```python
from build123d import *

# Parameters (mm, degrees)
SKETCH1_W           = 140
SKETCH1_H           = 25
BOSS_EXTRUDE1_DEPTH = 25
CUT_EXTRUDE1_DEPTH  = 25
CUT_EXTRUDE13_DEPTH = 3
SKETCH9_W           = 80
SKETCH9_H           = 18.70062617
CUT_EXTRUDE14_DEPTH = 3


with BuildPart() as part:
    # Sketch1 → Boss-Extrude1 (new body)
    with BuildSketch(Plane(origin=(0, 0, 0), x_dir=(1, 0, 0), z_dir=(0, 1, 0))):
        Rectangle(SKETCH1_W, SKETCH1_H)
    extrude(amount=BOSS_EXTRUDE1_DEPTH)

    # Sketch5 → Cut-Extrude1 (cut)
    with BuildSketch(Plane.XY.offset(12.5)):
        with BuildLine():
            add(Edge.make_bspline(
                [(0, 23), (15, 23), (30, 23.367346939)],
                knots=[0.5, 0.5, 0.5, 0.714285714, 0.714285714, 0.714285714], degree=2))
            add(Edge.make_bspline(
                [(30, 23.367346939), (50, 23.857142857), (70, 25)],
                knots=[0.714285714, 0.714285714, 0.714285714, 1, 1, 1], degree=2))
            Line((70, 25), (30, 25))
            Line((30, 25), (0, 25))
            Line((0, 25), (0, 23))
        make_face()
        with BuildLine():
            add(Edge.make_bspline(
                [(-50, 24.020408163), (-25, 23), (0, 23)],
                knots=[0.142857143, 0.142857143, 0.142857143, 0.5, 0.5, 0.5], degree=2))
            Line((0, 23), (0, 25))
            Line((0, 25), (-50, 25))
            Line((-50, 25), (-70, 25))
            add(Edge.make_bspline(
                [(-70, 25), (-60, 24.428571429), (-50, 24.020408163)],
                knots=[0, 0, 0, 0.142857143, 0.142857143, 0.142857143], degree=2))
        make_face()
        with BuildLine():
            Line((30, 19.867346939), (30, 23.367346939))
            add(Edge.make_bspline(
                [(0, 23), (15, 23), (30, 23.367346939)],
                knots=[0.5, 0.5, 0.5, 0.714285714, 0.714285714, 0.714285714], degree=2))
            Line((0, 23), (0, 19.5))
            add(Edge.make_bspline(
                [(0, 19.5), (14.999250637, 19.500030588), (30, 19.867346939)],
                knots=[0.625031228, 0.625031228, 0.625031228, 1, 1, 1], degree=2))
        make_face()
        with BuildLine():
            Line((0, 19.5), (0, 23))
            add(Edge.make_bspline(
                [(-50, 24.020408163), (-25, 23), (0, 23)],
                knots=[0.142857143, 0.142857143, 0.142857143, 0.5, 0.5, 0.5], degree=2))
            Line((-50, 24.020408163), (-50, 21.5))
            Line((-50, 21.5), (-50, 20.520408163))
            add(Edge.make_bspline(
                [(-50, 20.520408163), (-25.002082119, 19.499949013), (0, 19.5)],
                knots=[0, 0, 0, 0.625031228, 0.625031228, 0.625031228], degree=2))
        make_face()
        with BuildLine():
            Line((0, 0), (0, 3.5))
            add(Edge.make_bspline(
                [(-50, 4.813033374), (-25.004215516, 3.554754755), (0, 3.5)],
                knots=[0, 0, 0, 0.625063216, 0.625063216, 0.625063216], degree=2))
            Line((-50, 4.813033374), (-50, 1.020408163))
            add(Edge.make_bspline(
                [(-50, 1.020408163), (-25, 0), (0, 0)],
                knots=[0.142857143, 0.142857143, 0.142857143, 0.5, 0.5, 0.5], degree=2))
        make_face()
        with BuildLine():
            Line((30, 0.367346939), (30, 3.867346939))
            add(Edge.make_bspline(
                [(0, 3.5), (14.998483233, 3.467156007), (30, 3.867346939)],
                knots=[0.625063216, 0.625063216, 0.625063216, 1, 1, 1], degree=2))
            Line((0, 3.5), (0, 0))
            add(Edge.make_bspline(
                [(0, 0), (15, 0), (30, 0.367346939)],
                knots=[0.5, 0.5, 0.5, 0.714285714, 0.714285714, 0.714285714], degree=2))
        make_face()
        with BuildLine():
            Line((70, 0), (70, 2))
            add(Edge.make_bspline(
                [(30, 0.367346939), (50, 0.857142857), (70, 2)],
                knots=[0.714285714, 0.714285714, 0.714285714, 1, 1, 1], degree=2))
            add(Edge.make_bspline(
                [(0, 0), (15, 0), (30, 0.367346939)],
                knots=[0.5, 0.5, 0.5, 0.714285714, 0.714285714, 0.714285714], degree=2))
            Line((0, 0), (70, 0))
        make_face()
        with BuildLine():
            Line((-70, 0), (0, 0))
            add(Edge.make_bspline(
                [(-50, 1.020408163), (-25, 0), (0, 0)],
                knots=[0.142857143, 0.142857143, 0.142857143, 0.5, 0.5, 0.5], degree=2))
            add(Edge.make_bspline(
                [(-70, 2), (-60, 1.428571429), (-50, 1.020408163)],
                knots=[0, 0, 0, 0.142857143, 0.142857143, 0.142857143], degree=2))
            Line((-70, 2), (-70, 0))
        make_face()
    extrude(amount=-CUT_EXTRUDE1_DEPTH, mode=Mode.SUBTRACT)

    # Sketch6 → Cut-Extrude13 (cut)
    with BuildSketch(Plane.XY.offset(12.5)):
        with BuildLine():
            Line((30, 1.485887188), (30, 3.867346939))
            add(Edge.make_bspline(
                [(-50, 4.813033374), (-10.010789538, 2.799991192), (30, 3.867346939)],
                knots=[0, 0, 0, 1, 1, 1], degree=2))
            Line((-50, 4.813033374), (-50, 1.485887188))
            Line((-50, 1.485887188), (30, 1.485887188))
        make_face()
        with BuildLine():
            Line((-50, 20.520408163), (-50, 4.813033374))
            add(Edge.make_bspline(
                [(-50, 4.813033374), (-10.010789538, 2.799991192), (30, 3.867346939)],
                knots=[0, 0, 0, 1, 1, 1], degree=2))
            Line((30, 3.867346939), (30, 19.867346939))
            add(Edge.make_bspline(
                [(30, 19.867346939), (-10.005329691, 18.887755097), (-50, 20.520408163)],
                knots=[0, 0, 0, 1, 1, 1], degree=2))
        make_face()
        Polygon((-50, 20.520408163), (30, 19.867346939), (30, 20.995155466), (30, 21.46990277), (-50, 21.46990277), align=None)
        with BuildLine():
            Line((-50, 20.520408163), (30, 19.867346939))
            add(Edge.make_bspline(
                [(30, 19.867346939), (-10.005329691, 18.887755097), (-50, 20.520408163)],
                knots=[0, 0, 0, 1, 1, 1], degree=2))
        make_face()
    extrude(amount=-CUT_EXTRUDE13_DEPTH, mode=Mode.SUBTRACT)

    # Sketch9 → Cut-Extrude14 (cut)
    with BuildSketch(Plane(origin=(0, 0, -12.5), x_dir=(-1, 0, 0), z_dir=(0, 0, -1))):
        with Locations((10, 12.267033854)):
            Rectangle(SKETCH9_W, SKETCH9_H)
    extrude(amount=-CUT_EXTRUDE14_DEPTH, mode=Mode.SUBTRACT)


solid = part.part
```
Geometry: final body of the model. Coordinates: model frame, mm. A direction names the side the tool comes from. Give positions to 0.01 mm unless a question says otherwise; leave off trailing zeros. Loops run counter-clockwise (first coordinate to the right, second up) from the corner with the lowest first, then second, coordinate; pieces in that order, holes last. Notation, with made-up numbers: (75.5, 85) -> (104.5, 85) arc R22 ccw to (104.5, 98) -> close; hole circle Ø10 at (63, -36). An arc over 180 degrees is marked (long way). Return JSON: item names as keys, results as strings.
Item 1: Mould query, pull axis X, two halves, no side actions, for faces 4 (the flat face through (-60, 13, 12.5)), 5 (the flat face through (-11, 12, 9.5)), 6 (the flat face through (70, 13, 0)), 7 (the flat face through (-70, 13, 0)). Classes: released by +X, released by -X, zero draft, split by the parting line, or undercut.
Filled in:
{"face 4": "zero draft", "face 5": "undercut", "face 6": "released by +X", "face 7": "released by -X"}
Item 2: Section A-A, the plane y = 17.5. Output: boundary loops of the cut face in (x, z), plus the area to 3 significant figures.
Filled in:
{"outline": "(-70, -12.5) -> (-50, -12.5) -> (-50, -9.5) -> (30, -9.5) -> (30, -12.5) -> (70, -12.5) -> (70, 12.5) -> (30, 12.5) -> (30, 9.5) -> (-50, 9.5) -> (-50, 12.5) -> (-70, 12.5) -> close", "area": "3,020 mm^2"}
Item 3: Line query: line 1 (X direction, y = 22.75, z = -0.75); line 2 (Z direction, x = -13, y = 13); line 3 (Y direction, x = 6.5, z = 5.5). Output: solid intervals per line, ascending.
Filled in:
{"line 1": "-70 to -50, 30 to 70", "line 2": "-9.5 to 9.5", "line 3": "3.51 to 19.52"}
Item 4: Access query for faces 1 (the flat face through (50, 13, 12.5)), 2 (the flat face through (-50, 23, 0)), 3 (the flat face through (-9, 12, -9.5)). Directions: +Z, -Z, +X, -X, +Y, -Y. A direction counts if a zero-diameter tool reaches every point of the face in a straight line with its end or side. Return the directions, or none.
Filled in:
{"face 1": "+Z, +X, -X, +Y, -Y", "face 2": "none", "face 3": "-Z, +Y, -Y"}
Item 5: Pin query (flat end, axial travel): P1, Ø1.5, axis at x = -12.5, y = 7, coming from the -Z side; P2, Ø1.5, axis at x = -10.5, z = 3.5, coming from the -Y side; P3, Ø5, axis at x = -22.5, z = 5, coming from the +Y side. Return the tip coordinate at first contact, or that it passes through.
Filled in:
{"P1": "z = -9.5", "P2": "y = 3.57", "P3": "y = 19.76"}
